```python
from build123d import *

# Parameters (mm, degrees)
SKETCH3_W           = 148
SKETCH3_H           = 60
SKETCH3_R           = 15.1
SKETCH3_R_2         = 14.05
BOSS_EXTRUDE2_DEPTH = 3
FILLET1_R           = 4
EVK4_HOLES_D        = 2.15
FLIR_HOLES_D        = 3.2
VN_MOUNT_HOLES_D    = 3.175
VN_REF_HOLES_D      = 1.55
PCB_MOUNT_HOLES_D   = 3.2


with BuildPart() as part:
    # Sketch3 → Boss-Extrude2 (new body)
    with BuildSketch(Plane.XY):
        Rectangle(SKETCH3_W, SKETCH3_H)
        with Locations((-35, 0)):
            Circle(SKETCH3_R, mode=Mode.SUBTRACT)
        with Locations((35, 0)):
            Circle(SKETCH3_R_2, mode=Mode.SUBTRACT)
    extrude(amount=-BOSS_EXTRUDE2_DEPTH)

    # Fillet1
    fillet1_edges = [part.edges().sort_by_distance(p)[0] for p in [
        (-74, 30, -1.5),
        (74, 30, -1.5),
        (74, -30, -1.5),
        (-74, -30, -1.5),
    ]]
    fillet(fillet1_edges, radius=FILLET1_R)

    # EVK4-Holes (through all)
    with Locations(Plane.XY):
        with Locations((-47.5, 12.5), (-22.5, 12.5), (-22.5, -12.5), (-47.5, -12.5)):
            Hole(EVK4_HOLES_D / 2)

    # FLIR-Holes (through all)
    with Locations(Plane.XY):
        with Locations((15.5, 19.5), (54.5, 19.5), (54.5, -19.5), (15.5, -19.5)):
            Hole(FLIR_HOLES_D / 2)

    # VN-Mount-Holes (through all)
    with Locations(Plane.XY):
        with Locations((-15.42, -3.81), (15.4159, -3.81)):
            Hole(VN_MOUNT_HOLES_D / 2)

    # VN-Ref-Holes (through all)
    with Locations(Plane.XY):
        with Locations((-15.42, 0), (15.4159, 0)):
            Hole(VN_REF_HOLES_D / 2)

    # PCB-Mount-Holes (through all)
    with Locations(Plane.XY):
        with Locations((-22.4, 26), (19.6, 26), (19.6, -26), (-22.4, -26)):
            Hole(PCB_MOUNT_HOLES_D / 2)


solid = part.part
```
Input: part model. Units: mm. Frame: model coordinates. Round coordinates to 2 decimals unless told otherwise and drop trailing zeros. Order: outer loops, then holes, each group sorted by start corner. A loop starts at its lowest first (then second) coordinate and runs counter-clockwise, first axis right, second up. Notation, with made-up numbers: (73.25, 3) - (89.25, 3) arc R36 cw to (89.25, 40) - close; hole circle Ø3 at (68, 61.25). An arc over 180 degrees is marked (long way). One line per question, with ' | ' between items. Start each with the question number.
1) Cut plane D-D, the plane y = 3.5. Return the cut outline in (x, z), then the cut area to 3 significant figures.
2) Cut plane B-B, the plane x = 35. Return the cut outline in (y, z), then the cut area to 3 significant figures.
3) Cut plane C-C, the plane z = -0.95. Give the number of separate pieces and of enclosed holes in the cut face, then the cut area to 3 significant figures.
4) Cut plane A-A, the plane y = -19.5. Return the cut outline in (x, z).
5) Pull-direction query (Y, two-part tool) for faces 1 (the flat face through (-1, 30, -1)), 2 (the flat face through (-1, 0, -3)), 3 (the cylindrical face through (-16.934, -3.333, -1.521)), 4 (the cylindrical face through (-24, -26, -2)); classes: +Y half, -Y half, draft (parallel to the pull), parting line (faces both ways), or undercut.
6) Ray query, probe 1 along Y at (x, z) = (54.5, -1.75); probe 2 along X at (y, z) = (-9, -0.65); probe 3 along X at (y, z) = (3.5, -1.15). Return the intervals inside material, ascending.
Worked out:
1) outline: (-74, -3) - (-49.69, -3) - (-49.69, 0) - (-74, 0) - close; (-20.31, -3) - (21.39, -3) - (21.39, 0) - (-20.31, 0) - close; (48.61, -3) - (74, -3) - (74, 0) - (48.61, 0) - close | area: 274 mm^2
2) outline: (-30, -3) - (-14.05, -3) - (-14.05, 0) - (-30, 0) - close; (14.05, -3) - (30, -3) - (30, 0) - (14.05, 0) - close | area: 95.7 mm^2
3) separate pieces: 1 | enclosed holes: 18 | area: 7,430 mm^2
4) outline: (-74, -3) - (13.9, -3) - (13.9, 0) - (-74, 0) - close; (17.1, -3) - (52.9, -3) - (52.9, 0) - (17.1, 0) - close; (56.1, -3) - (74, -3) - (74, 0) - (56.1, 0) - close
5) face 1: +Y half | face 2: draft | face 3: undercut | face 4: undercut
6) probe 1: y = -30 to -21.1, -17.9 to 17.9, 21.1 to 30 | probe 2: x = -74 to -47.12, -22.88 to 24.21, 45.79 to 74 | probe 3: x = -74 to -49.69, -20.31 to 21.39, 48.61 to 74
